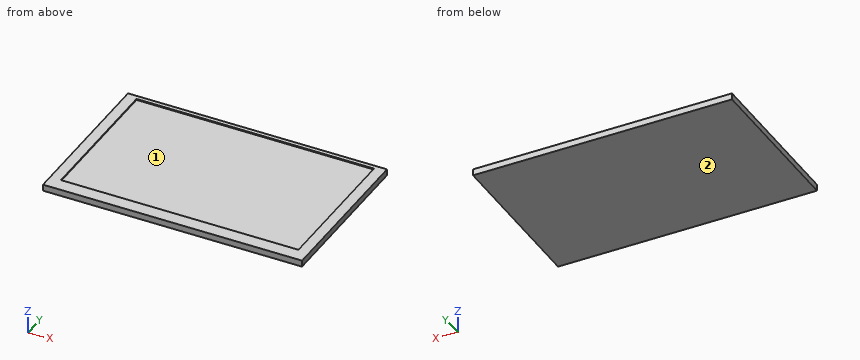
Autodesk Fusion 360 part; units mm, degrees
sketch "Sketch1" plane through (0, 0, 0) normal (0, 0, 1) x (1, 0, 0)
  line L0 (0, 0) -> (120.7, 0)
  line L1 (120.7, 0) -> (120.7, 75.8)
  line L2 (120.7, 75.8) -> (0, 75.8)
  line L3 (0, 75.8) -> (0, 0)
  line L4 (5, 73.8) -> (115.7, 73.8)
  line L5 (115.7, 73.8) -> (115.7, 6.4)
  line L6 (115.7, 6.4) -> (5, 6.4)
  line L7 (5, 6.4) -> (5, 73.8)
  dimension "d1" = 120.7
  dimension "d2" = 75.8
  dimension "d3" = 2
  dimension "d4" = 6.4
  dimension "d5" = 5
  dimension "d6" = 5
extrude "Extrude1" add sketch "Sketch1" along normal blind 3 contours L0 L1 L2 L3 | L4 L5 L6 L7
extrude "Extrude2" cut sketch "Sketch1" along normal blind 0.5 from surface at 2.5 contours L4 L5 L6 L7
Work out the finished part from the listing and answer in its coordinate system (mm). Face numbers are marked on the shaded views. Round coordinates to 2 decimals unless told otherwise and drop trailing zeros. Write each loop counter-clockwise with the first axis right and the second up, starting at its lowest first coordinate (ties: lowest second). Pieces come first, ordered by that corner, then holes.
1) A cutting plane is placed at A-A on y = 34. Determine the outline of the cut face in (x, z).
2) Determine the mould class of the marked faces 1 and 2 for opening direction X: pulls with the +X half, pulls with the -X half, needs draft (parallel to the pull), parting line crosses it, or undercut.
3) A cutting plane is placed at B-B on x = 57. Determine the outline of the cut face in (y, z).
4) Consider probe 1 along X at (y, z) = (61, 2.7); probe 2 along Z at (x, y) = (110.5, 11.5). Determine where each line is inside the solid, lowest interval first.
Entries:
1. outline: (0, 0) - (120.7, 0) - (120.7, 3) - (115.7, 3) - (115.7, 2.5) - (5, 2.5) - (5, 3) - (0, 3) - close
2. face 1: undercut
2. face 2: needs draft
3. outline: (0, 0) - (75.8, 0) - (75.8, 3) - (73.8, 3) - (73.8, 2.5) - (6.4, 2.5) - (6.4, 3) - (0, 3) - close
4. probe 1: x = 0 to 5, 115.7 to 120.7
4. probe 2: z = 0 to 2.5
